Check sheet for the modelled part. Datum: model origin and axes. Units: mm. Give positions to 0.01 mm unless a question says otherwise; leave off trailing zeros. Order: outer loops, then holes, each group sorted by start corner. A loop starts at its lowest first (then second) coordinate and runs counter-clockwise, first axis right, second up. Notation, with made-up numbers: M 6.25,55.5 L 40.25,55.5 A11 cw 40.25,70.5 Z; hole C -37,-3 d11. An arc over 180 degrees is marked long. Answer in a Markdown table with one row per item. Add a question column.
from build123d import *

# Parameters (mm, degrees)
SKETCH1_W           = 6
SKETCH1_H           = 5
BOSS_EXTRUDE1_DEPTH = 0.5
SKETCH2_W           = 7
SKETCH2_H           = 5
BOSS_EXTRUDE2_DEPTH = 4.5
SKETCH3_R           = 0.8
CUT_EXTRUDE1_DEPTH  = 9.958236434
CHAMFER1_SIZE       = 0.5


with BuildPart() as part:
    # Sketch1 → Boss-Extrude1 (new body)
    with BuildSketch(Plane(origin=(0, 0, 0), x_dir=(1, 0, 0), z_dir=(0, 1, 0))):
        Rectangle(SKETCH1_W, SKETCH1_H)
    extrude(amount=BOSS_EXTRUDE1_DEPTH)

    # Sketch2 → Boss-Extrude2 (add)
    with BuildSketch(Plane(origin=(0, 0.5, 0), x_dir=(1, 0, 0), z_dir=(0, 1, 0))):
        Rectangle(SKETCH2_W, SKETCH2_H)
    extrude(amount=BOSS_EXTRUDE2_DEPTH)

    # Sketch3 → Cut-Extrude1 (cut, through all)
    with BuildSketch(Plane.ZY.offset(3.5)):
        with Locations((0, 1.58)):
            Circle(SKETCH3_R)
    extrude(amount=-CUT_EXTRUDE1_DEPTH, mode=Mode.SUBTRACT)

    # Chamfer1
    # the kernel refuses this chamfer: 0.5 mm, written as the material it takes off along each edge
    with BuildSketch(Plane(origin=(3.5, 1.58, 0), x_dir=(0, 0, 1), z_dir=(0, -1, 0))) as chamfer1_piece_1:
        Polygon((0.8 + CHAMFER1_SIZE, 0), (0.8, CHAMFER1_SIZE), (0.8, 0), align=None)
    revolve(axis=Axis((3.5, 1.58, 0), (-1, 0, 0)), mode=Mode.SUBTRACT)
    with BuildSketch(Plane(origin=(-3.5, 1.58, 0), x_dir=(0, 0, 1), z_dir=(0, -1, 0))) as chamfer1_piece_2:
        Polygon((0.8 + CHAMFER1_SIZE, 0), (0.8, -CHAMFER1_SIZE), (0.8, 0), align=None)
    revolve(axis=Axis((-3.5, 1.58, 0), (-1, 0, 0)), mode=Mode.SUBTRACT)


solid = part.part
Q1. Cross-section at A-A (y = 1.58). Record the boundary of the cut face in (x, z).
Q2. Draft check along Y on faces 1 (the cylindrical face through (-0.042, 2.373, -0.104)), 2 (the flat face through (0, 0, 0)), 3 (the flat face through (0, 5, 0)), 4 (the flat face through (-3.5, 3.2, 0)). Enter one of: pulls with the +Y half, pulls with the -Y half, needs draft (parallel to the pull), parting line crosses it, or undercut.
Q3. Go/stop test with flat-tipped pins: pin 1 (1 mm diameter, centred on y = 1.58, z = 0, fed in from +X); pin 2 (0.6 mm diameter, centred on x = 3.5, z = 0.5, fed in from -Y). Record where each tip stops, or that it passes through.
Q4. Thickness scan on probe 1 along Y at (x, z) = (-0.55, 0); probe 2 along Z at (x, y) = (0.75, 0.95); probe 3 along Y at (x, z) = (-2.25, 0.6). Record the ranges inside material, lowest first.
Q5. Cross-section at B-B (z = 0). Record the boundary of the cut face in (x, y).
Q6. Cross-section at C-C (x = -2.25). Record the boundary of the cut face in (y, z).
Values follow:
| question | item | result |
|---|---|---|
| 1 | outline | M -3.5,-2.5 L 3.5,-2.5 L 3.5,-1.3 L 3,-0.8 L -3,-0.8 L -3.5,-1.3 Z; M -3.5,1.3 L -3,0.8 L 3,0.8 L 3.5,1.3 L 3.5,2.5 L -3.5,2.5 Z |
| 2 | face 1 | undercut |
| 2 | face 2 | pulls with the -Y half |
| 2 | face 3 | pulls with the +Y half |
| 2 | face 4 | needs draft |
| 3 | pin 1 | through |
| 3 | pin 2 | y = 0.5 |
| 4 | probe 1 | 0 to 0.78, 2.38 to 5 |
| 4 | probe 2 | -2.5 to -0.49, 0.49 to 2.5 |
| 4 | probe 3 | 0 to 1.05, 2.11 to 5 |
| 5 | outline | M -3.5,2.88 L -3,2.38 L 3,2.38 L 3.5,2.88 L 3.5,5 L -3.5,5 Z; M -3.28,0.5 L -3,0.5 L -3,0 L 3,0 L 3,0.5 L 3.28,0.5 L 3,0.78 L -3,0.78 Z |
| 6 | outline | M 0,-2.5 L 5,-2.5 L 5,2.5 L 0,2.5 Z; hole C 1.58,0 d1.6 |
